The listing builds one solid part. Answer for the finished solid, in the listing's coordinates (mm). Face numbers are marked on the shaded views. Coordinates: 2 decimals unless noted, no trailing zeros. Loops run counter-clockwise (first coordinate to the right, second up) from the corner with the lowest first, then second, coordinate; pieces in that order, holes last. Notation, with made-up numbers: M -36,-35.5 L 18,-35.5 A24 ccw 18,-18.5 Z; hole C 1,17 d4. An arc over 180 degrees is marked long. Answer as CSV lines item,"result". Start each with the question number.
Autodesk Inventor part; units mm, degrees
ref_plane "YZ Plane" through (0, 0, 0) normal (1, 0, 0) x (0, 1, 0)
ref_plane "XZ Plane" through (0, 0, 0) normal (0, 1, 0) x (-1, 0, 0)
ref_plane "XY Plane" through (0, 0, 0) normal (0, 0, 1) x (1, 0, 0)
sketch "Sketch1" plane through (0, 0, 0) normal (0, 0, 1) x (1, 0, 0)
  line L0 (-10.4625, 19.3656) -> (31.5375, 19.3656)
  line L1 (31.5375, 19.3656) -> (31.5375, -2.6344)
  line L2 (31.5375, -2.6344) -> (-10.4625, -2.6344)
  line L3 (-10.4625, -2.6344) -> (-10.4625, 19.3656)
  point P0 (0, 0)
  dimension "d0" = 42
  dimension "d1" = 22
extrude "Extrusion1" add sketch "Sketch1" along normal blind 10
sketch "Sketch2" plane through (0, 0, 10) normal (0, 0, 1) x (1, 0, 0)
  line L0 (-10.4625, -2.6344) -> (31.5375, -2.6344)
  arc A0 (0.0751, -2.6344) -> (0.0375, 4.3656) centre (0.0751, 0.8657) ccw
  arc A1 (-0.0002, 11.3656) -> (0.0375, 4.3656) centre (-0.0002, 7.8655) ccw
  arc A2 (21.0375, 4.3656) -> (20.9998, -2.6344) centre (20.9998, 0.8657) ccw
  arc A3 (21.0375, 4.3656) -> (21.0751, 11.3656) centre (21.0751, 7.8655) ccw
  line L1 (-0.0002, 11.3656) -> (21.0751, 11.3656)
  line L2 (0.0751, 0.8657) -> (0.0375, 4.3656) construction
  line L3 (21.0751, 7.8655) -> (21.0375, 4.3656) construction
  line L4 (21.0375, 4.3656) -> (20.9998, 0.8657) construction
  line L5 (-10.4625, 19.3656) -> (-10.4625, -2.6344)
  line L6 (0.0375, 4.3656) -> (-0.0002, 7.8655) construction
  point P0 (0, 0)
  point P1 (10.5375, 11.3656)
  dimension "d4" = 21
  dimension "d5" = 21
  dimension "d6" = 14
extrude "Extrusion2" cut sketch "Sketch2" against normal through all
sketch "Sketch3" plane through (0, 0, 10) normal (0, 0, 1) x (1, 0, 0)
  line L0 (-0.0002, 11.3656) -> (21.0751, 11.3656)
  arc A0 (-0.0002, 11.3656) -> (9.5375, 17.3656) centre (-0.0002, 21.9462) ccw
  arc A1 (11.5375, 17.3656) -> (21.0751, 11.3656) centre (21.0751, 21.9462) ccw
  line L1 (9.5375, 17.3656) -> (11.5375, 17.3656)
  line L2 (31.5375, 19.3656) -> (-10.4625, 19.3656)
  arc A2 (21.0375, 4.3656) -> (21.0751, 11.3656) centre (21.0751, 7.8655) ccw
  line L3 (-0.0002, 11.3656) -> (21.0751, 11.3656)
  point P0 (0, 0)
  dimension "d9" = 2
  dimension "d10" = 2
extrude "Extrusion3" cut sketch "Sketch3" against normal through all
pattern_linear "Rectangular Pattern1" count 2 spacing 42 along (-1, 0, 0) of "Extrusion1", "Extrusion2", "Extrusion3"
sketch "Sketch4" plane through (0, 0, 10) normal (0, 0, 1) x (1, 0, 0)
  line L0 (31.5375, 19.3656) -> (-52.4625, 19.3656)
  line L1 (-30.4543, 19.3656) -> (-30.4543, -2.6344)
  line L2 (-52.4625, -2.6344) -> (-41.9249, -2.6344)
  line L3 (-30.4543, -2.6344) -> (-52.4625, -2.6344)
  line L4 (-52.4625, -2.6344) -> (-52.4625, 19.3656)
  line L5 (-52.4625, 19.3656) -> (-30.4543, 19.3656)
  line L6 (9.5367, 19.3656) -> (9.5367, -2.6344)
  line L7 (20.9998, -2.6344) -> (31.5375, -2.6344)
  line L8 (9.5367, -2.6344) -> (31.5375, -2.6344)
  line L9 (31.5375, -2.6344) -> (31.5375, 19.3656)
  line L10 (31.5375, 19.3656) -> (9.5367, 19.3656)
  point P0 (0, 0)
extrude "Extrusion4" cut sketch "Sketch4" against normal through all
sketch "Sketch5" plane through (0, 0, 10) normal (0, 0, 1) x (1, 0, 0)
  arc A0 (-20.9625, 4.3656) -> (-20.9249, 11.3656) centre (-20.9249, 7.8655) ccw
  line L0 (-20.9625, 4.3656) -> (-21.1286, -11.0791) construction
  arc A1 (-0.0002, 11.3656) -> (0.0375, 4.3656) centre (-0.0002, 7.8655) ccw construction
  line L1 (-20.9625, 4.3656) -> (-9.8965, 4.2466) construction
  line L2 (-20.9625, 4.3656) -> (-20.6751, 31.0931) construction
  arc A2 (0.0751, -2.6344) -> (0.0375, 4.3656) centre (0.0751, 0.8657) ccw
  arc A3 (-20.9625, 4.3656) -> (-21.0002, -2.6344) centre (-21.0002, 0.8657) ccw
  line L3 (9.5367, 19.3656) -> (-30.4543, 19.3656) construction
  line L4 (-10.4588, 19.3656) -> (-10.4625, -2.6344) construction
  line L5 (-21.0002, -2.6344) -> (0.0751, -2.6344) construction
  line L6 (0.0375, 4.3656) -> (-2.5475, 4.3378) construction
  line L7 (0.0375, 4.3656) -> (0.6415, 4.3721) construction
  line L8 (0.0375, 4.3656) -> (-0.1492, 21.7223) construction
  point P0 (0, 0)
  point P1 (-20.8344, 16.2756)
  point P2 (-0.0906, 16.2766)
hole "Hole1" at (-20.8344, 16.2756, 10) at (-0.0906, 16.2766, 10) direction (0, 0, -1) diameter 3 end through all
properties part number "Zipperteethv5"
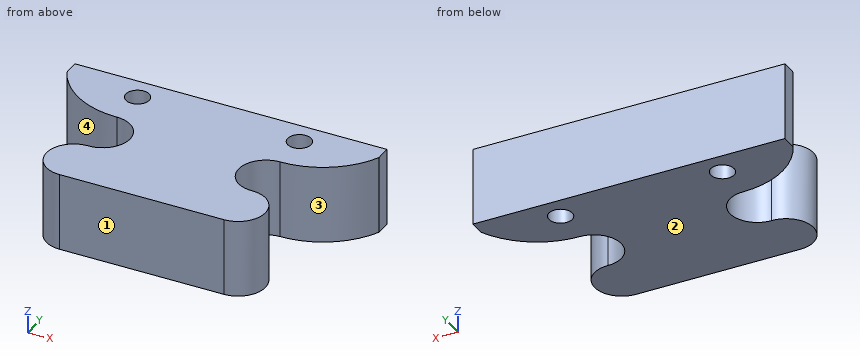
Item 1: Consider line 1 (Y direction, x = 0, z = 8.75); line 2 (X direction, y = 15.75, z = 1.25); line 3 (Y direction, x = 1, z = 3.75). Determine where each line is inside the solid, lowest interval first.
Item 2: For a pull along Y with two mould halves and no side action, classify the marked faces 1, 2, 3 and 4 as pulls with the +Y half, pulls with the -Y half, needs draft (parallel to the pull), parting line crosses it, or undercut.
Item 3: Section D-D on y = 8 is taken. Determine the outline of the cut face in (x, z), then the cut area to 3 significant figures.
Item 4: Each of these flat-tipped pins is pushed along its axis until it touches: P1, Ø1, axis at y = 9.5, z = 4.5, coming from the +X side; P2, Ø1.5, axis at y = 7, z = 3.5, coming from the -X side; P3, Ø1, axis at y = 14, z = 6, coming from the -X side. Where does it stop, or does it pass through?
Item 5: Section C-C on x = 4.5 is taken. Determine the outline of the cut face in (y, z), then the cut area to 3 significant figures.
Item 6: Section A-A on x = -2.5 is taken. Determine the outline of the cut face in (y, z), then the cut area to 3 significant figures.
Item 7: Section B-B on z = 5.75 is taken. Determine the outline of the cut face in (x, y), then the cut area to 3 significant figures.
Results are:
1,line 1,"-2.63 to 4.37, 11.37 to 14.78, 17.77 to 19.37"
1,line 2,"-29.5 to -22.24, -19.43 to -1.5, 1.31 to 8.58"
1,line 3,"-2.51 to 4.24, 11.41 to 15.25, 17.31 to 19.37"
2,face 1,"pulls with the -Y half"
2,face 2,"needs draft"
2,face 3,"undercut"
2,face 4,"undercut"
3,outline,"M -17.43,0 L -3.5,0 L -3.5,10 L -17.43,10 Z"
3,area,"139 mm²"
4,P1,"x = -2.77"
4,P2,"x = -17.82"
4,P3,"x = -28.44"
5,outline,"M 12.37,0 L 19.37,0 L 19.37,10 L 12.37,10 Z"
5,area,"70.0 mm²"
6,outline,"M -2.63,0 L 5.42,0 L 5.42,10 L -2.63,10 Z; M 10.32,0 L 19.37,0 L 19.37,10 L 10.32,10 Z"
6,area,"171 mm²"
7,outline,"M -30.45,17.35 A10.58 ccw -20.92,11.37 A3.5 cw long -20.96,4.37 A3.5 ccw long -21,-2.63 L 0.08,-2.63 A3.5 ccw long 0.04,4.37 A3.5 cw long 0,11.37 A10.58 ccw 9.54,17.36 L 9.54,19.37 L -30.45,19.37 Z; hole C -20.83,16.28 d3; hole C -0.09,16.28 d3"
7,area,"567 mm²"
